Read the model definition and answer for the solid it produces. Units are mm, in the model's axes. A direction names the side the tool comes from. Coordinates: 2 decimals unless noted, no trailing zeros. Write each loop counter-clockwise with the first axis right and the second up, starting at its lowest first coordinate (ties: lowest second). Pieces come first, ordered by that corner, then holes.
1) Find the intervals of material crossed by line 1 (X direction, y = -0.75, z = 11); line 2 (X direction, y = -9.5, z = 24.75); line 3 (Y direction, x = 13, z = 16), in increasing order.
2) Determine the mould class of faces 1 (the face through (52, 2, 15)), 2 (the face through (15.5, -2, 15)), 3 (the face through (17.359, 10.297, 14.79)) for opening direction Y: +Y half, -Y half, draft (parallel to the pull), parting line (faces both ways), or undercut.
3) The part is cut by section B-B (y = -2.5). Determine the outline of the cut face in (x, z).
4) Which of the six approach directions +Z, -Z, +X, -X, +Y, -Y give full straight-line access (tool end or side, diameter ignored) to faces 4 (the face through (49, 3, 15)), 5 (the face through (-18, -3, 15)), 6 (the face through (0, 8.5, 15)), 7 (the face through (-15, -3, 15)), 8 (the face through (18.5, -9, 15))?
5) The part is cut by section C-C (z = 17.5). Determine the outline of the cut face in (x, y), then the cut area to 3 significant figures.
6) Each of these flat-tipped pins is pushed along its axis until it touches: pin 1 Ø1.5 at (x, z) = (3, 16) entering from -Y; pin 2 Ø2 at (x, z) = (38, 24.5) entering from -Y; pin 3 Ø2.5 at (y, z) = (-10, 21.5) entering from +X. Where does it stop, or does it pass through?
7) The part is cut by section A-A (y = 4.5). Determine the outline of the cut face in (x, z).
8) The part is cut by section D-D (y = -9.5). Determine the outline of the cut face in (x, z).
from build123d import *

# Parameters (mm, degrees)
EXTRUDE_THIN1_DEPTH = 30
BOSS_EXTRUDE1_DEPTH = 30
SKETCH3_W           = 30
SKETCH3_H           = 3
EXTRUDE_THIN2_DEPTH = 30
BOSS_EXTRUDE2_DEPTH = 30


with BuildPart() as part:
    # Sketch1 → Extrude-Thin1 (new body)
    with BuildSketch(Plane.XY):
        with BuildLine():
            Line((-15, -12.5), (-15, 7.5))
            ThreePointArc((-15, 7.5), (-14.707106781, 8.207106781), (-14, 8.5))
            Line((-14, 8.5), (14.5, 8.5))
            ThreePointArc((14.5, 8.5), (15.207106781, 8.207106781), (15.5, 7.5))
            Line((15.5, 7.5), (15.5, -12.5))
            Line((15.5, -12.5), (18.5, -12.5))
            Line((18.5, -12.5), (18.5, 7.5))
            ThreePointArc((18.5, 7.5), (17.328427125, 10.328427125), (14.5, 11.5))
            Line((14.5, 11.5), (-14, 11.5))
            ThreePointArc((-14, 11.5), (-16.828427125, 10.328427125), (-18, 7.5))
            Line((-18, 7.5), (-18, -12.5))
            Line((-18, -12.5), (-15, -12.5))
        make_face()
    extrude(amount=EXTRUDE_THIN1_DEPTH)

    # Sketch2 → Boss-Extrude1 (add)
    with BuildSketch(Plane.XY.offset(30)):
        Polygon((-15, -13.5), (-18, -13.5), (-18, -12.5), (-15, -12.5), (-14.6, -12.7), align=None)
        Polygon((15.5, -12.5), (15.1, -12.7), (15.5, -13.5), (18.5, -13.5), (18.5, -12.5), align=None)
    extrude(amount=-BOSS_EXTRUDE1_DEPTH)

    # Sketch3 → Extrude-Thin2 (add)
    with BuildSketch(Plane(origin=(18.5, 0, 0), x_dir=(0, 0, -1), z_dir=(1, 0, 0))):
        with Locations((-15, -3)):
            Rectangle(SKETCH3_W, SKETCH3_H)
    extrude(amount=EXTRUDE_THIN2_DEPTH)

    # Sketch4 → Boss-Extrude2 (add)
    with BuildSketch(Plane.XY.offset(30)):
        with BuildLine():
            Line((48.5, -1.5), (49, -1.5))
            Line((49, -1.5), (49, 7.5))
            ThreePointArc((49, 7.5), (49.292893219, 8.207106781), (50, 8.5))
            Line((50, 8.5), (51, 8.5))
            ThreePointArc((51, 8.5), (51.707106781, 8.207106781), (52, 7.5))
            Line((52, 7.5), (52, -3.5))
            ThreePointArc((52, -3.5), (51.707106781, -4.207106781), (51, -4.5))
            Line((51, -4.5), (48.5, -4.5))
            Line((48.5, -4.5), (48.5, -1.5))
        make_face()
    extrude(amount=-BOSS_EXTRUDE2_DEPTH)


solid = part.part
Reported:
1. line 1: x = -18 to -15, 15.5 to 18.5, 49 to 52
1. line 2: x = -18 to -15, 15.5 to 18.5
1. line 3: y = 8.5 to 11.5
2. face 1: draft
2. face 2: undercut
2. face 3: +Y half
3. outline: (-18, 0) - (-15, 0) - (-15, 30) - (-18, 30) - close; (15.5, 0) - (52, 0) - (52, 30) - (15.5, 30) - close
4. face 4: +Z, -Z, +Y
4. face 5: +Z, -Z, -X, +Y, -Y
4. face 6: +Z, -Z, -Y
4. face 7: +Z, -Z
4. face 8: +Z, -Z, +X, -Y
5. outline: (-18, -13.5) - (-15, -13.5) - (-14.6, -12.7) - (-15, -12.5) - (-15, 7.5) arc R1 cw to (-14, 8.5) - (14.5, 8.5) arc R1 cw to (15.5, 7.5) - (15.5, -12.5) - (15.1, -12.7) - (15.5, -13.5) - (18.5, -13.5) - (18.5, -4.5) - (51, -4.5) arc R1 ccw to (52, -3.5) - (52, 7.5) arc R1 ccw to (51, 8.5) - (50, 8.5) arc R1 ccw to (49, 7.5) - (49, -1.5) - (18.5, -1.5) - (18.5, 7.5) arc R4 ccw to (14.5, 11.5) - (-14, 11.5) arc R4 ccw to (-18, 7.5) - close
5. area: 365 mm2
6. pin 1: stops at y = 8.5
6. pin 2: stops at y = -4.5
6. pin 3: stops at x = 18.5
7. outline: (-18, 0) - (-15, 0) - (-15, 30) - (-18, 30) - close; (15.5, 0) - (18.5, 0) - (18.5, 30) - (15.5, 30) - close; (49, 0) - (52, 0) - (52, 30) - (49, 30) - close
8. outline: (-18, 0) - (-15, 0) - (-15, 30) - (-18, 30) - close; (15.5, 0) - (18.5, 0) - (18.5, 30) - (15.5, 30) - close
